```python
from build123d import *

# Parameters (mm, degrees)
SKETCH2_W          = 8
SKETCH2_H          = 8
CUT_EXTRUDE1_DEPTH = 76


with BuildPart() as part:
    # Sketch1 → Revolve1 (revolve)
    with BuildSketch(Plane.XY):
        Polygon((75, -15), (10, -15), (0, -70), (0, -75), (10, -75), (16.659953574, -65), (21.299953574, -65), (26.250205442, -75), (36.250205442, -75), (40.571282755, -65), (45.211282755, -65), (52.646188266, -75), (62.646188266, -75), (62.646188266, -50), (75, -50), align=None)
    revolve(axis=Axis((0, 0, 0), (1, 0, 0)))

    # Sketch2 → Cut-Extrude1 (cut, through all)
    with BuildSketch(Plane(origin=(75, 0, 0), x_dir=(0, 0, -1), z_dir=(1, 0, 0))):
        with Locations((0, -15)):
            Rectangle(SKETCH2_W, SKETCH2_H)
    extrude(amount=-CUT_EXTRUDE1_DEPTH, mode=Mode.SUBTRACT)


solid = part.part
```
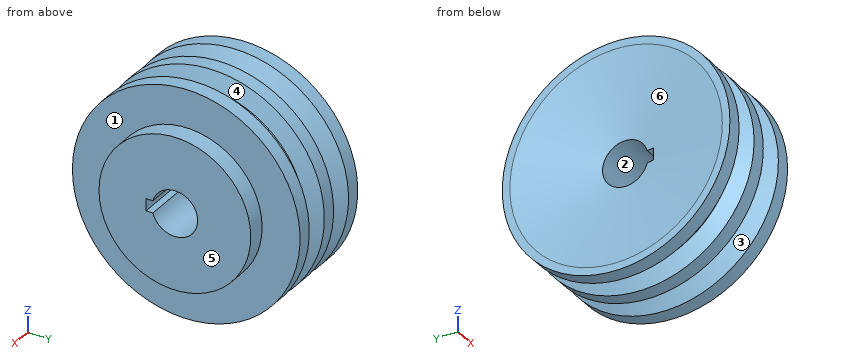
The model under review builds one solid part; all positions refer to its coordinate system, in mm. Face numbers are marked on the shaded views. A direction names the side the tool comes from. Round coordinates to 2 decimals unless told otherwise and drop trailing zeros. Loops run counter-clockwise (first coordinate to the right, second up) from the corner with the lowest first, then second, coordinate; pieces in that order, holes last. Notation, with made-up numbers: M -14.75,51 L -5.75,51 A24 ccw -5.75,61 Z; hole C -2.75,20.25 d10. An arc over 180 degrees is marked long. Write item = value, one per line.
Item 1: Insertion check: P1, Ø2, axis at y = -34.5, z = -18, coming from the -X side; P2, Ø2, axis at x = 64.5, z = -1.5, coming from the -Y side; P3, Ø6, axis at x = 14, y = -48.5, coming from the +Z side. Each pin has a flat end and moves straight along its axis. Give the tip position at first contact, or say it passes through.
Return value:
P1 = 5.47
P2 = -50
P3 = 55.76
Item 2: Machinability: for the marked faces 1, 2 and 3, which of the approach directions +Z, -Z, +X, -X, +Y, -Y give a long, thin tool a straight path to every point of the face, cutting with its end or side? Answer none if there is none.
Return value:
face_1 = +X
face_2 = +X, -X
face_3 = none
Item 3: For line 1 (X direction, y = -23, z = 68); line 2 (Z direction, x = 61, y = 0); line 3 (X direction, y = -64, z = 34), list the stretches that pass through material, from the lowest coordinate up. Write a range as [from, to].
Return value:
line_1 = [0, 12.14], [24.66, 37.64], [50.26, 62.65]
line_2 = [-75, -15], [15, 75]
line_3 = [0, 11.68], [25, 37.34], [50.77, 62.65]
Item 4: The part is to be moulded in two halves that separate along Y. For the marked faces 4, 5 and 6, say which applies: released by +Y, released by -Y, zero draft, split by the parting line, or undercut.
Return value:
face_4 = split by the parting line
face_5 = zero draft
face_6 = undercut
Item 5: Take a section at C-C on x = 6.5. Write out the cut boundary in (y, z), then the cut area to 3 significant figures.
Return value:
outline = C 0,0 d150; hole C 0,0 d68.5
area = 14,000 mm2
